Read the model definition and answer for the solid it produces. Units are mm, in the model's axes. Face numbers are marked on the shaded views. Give positions to 0.01 mm unless a question says otherwise; leave off trailing zeros. Loops run counter-clockwise (first coordinate to the right, second up) from the corner with the lowest first, then second, coordinate; pieces in that order, holes last. Notation, with made-up numbers: (49, 59.25) -> (77, 59.25) arc R21 cw to (77, 93.25) -> close; hole circle Ø11 at (86.25, 31.5). An arc over 180 degrees is marked (long way). Return JSON: item names as keys, results as strings. Group by question number.
Autodesk Inventor part; units mm, degrees
ref_plane "YZ Plane" through (0, 0, 0) normal (1, 0, 0) x (0, 1, 0)
ref_plane "XZ Plane" through (0, 0, 0) normal (0, 1, 0) x (-1, 0, 0)
ref_plane "XY Plane" through (0, 0, 0) normal (0, 0, 1) x (1, 0, 0)
sketch "Sketch1" plane through (0, 0, 0) normal (0, 0, 1) x (1, 0, 0)
  line L0 (0, 23.5) -> (3, 23.5)
  line L1 (5, 25.5) -> (5, 29.2)
  line L2 (5, 29.2) -> (10, 29.2)
  line L3 (10, 29.2) -> (10, 31.5)
  line L4 (10, 31.5) -> (0, 31.5)
  line L5 (0, 23.5) -> (0, 39.7331)
  arc A0 (3, 23.5) -> (5, 25.5) centre (3, 25.5) ccw
  line L6 (0, 0) -> (48.7382, 0)
  line L7 (0, 23.5) -> (-3, 23.5)
  line L8 (-5, 25.5) -> (-5, 29.2)
  line L9 (-5, 29.2) -> (-10, 29.2)
  line L10 (-10, 29.2) -> (-10, 31.5)
  line L11 (-10, 31.5) -> (0, 31.5)
  arc A1 (-5, 25.5) -> (-3, 23.5) centre (-3, 25.5) ccw
  dimension "d0" = 2
  dimension "d1" = 47
  dimension "d2" = 63
  dimension "d3" = 58.4
  dimension "d4" = 10
  dimension "d7" = 10
revolve "Revolution1" add sketch "Sketch1" angle 360 about axis through (0, 0, 0) along (1, 0, 0)
chamfer "Fase1" distance 1 angle 45 1 edges at (10, -29.2, 0)
chamfer "Fase2" distance 1 angle 45 1 edges at (-10, -29.2, 0)
properties part number "Plunger_Seal" material "Nylon-6/6"
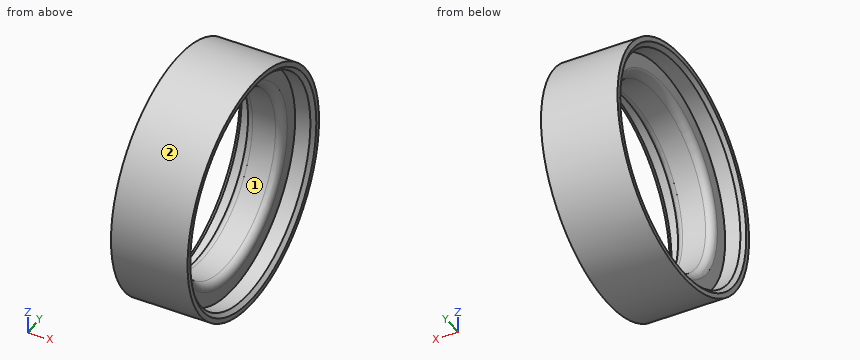
1. Section D-D on x = -7.5 is taken. Determine the outline of the cut face in (y, z), then the cut area to 3 significant figures.
2. Flat-ended cylindrical pins translate along their axes: pin 1 Ø8 at (x, z) = (-7.5, -25) entering from -Y; pin 2 Ø17.5 at (y, z) = (-12.5, -9) entering from +X; pin 3 Ø3 at (x, y) = (-7, -7.5) entering from +Z; pin 4 Ø2 at (y, z) = (-17.5, -14) entering from +X. Find the tip coordinate at first contact, or state that the pin passes through.
3. Determine the mould class of the marked faces 1 and 2 for opening direction Z: pulls with the +Z half, pulls with the -Z half, needs draft (parallel to the pull), parting line crosses it, or undercut.
4. Section A-A on z = 0 is taken. Determine the outline of the cut face in (x, y), then the cut area to 3 significant figures.
5. Section C-C on x = -2 is taken. Determine the outline of the cut face in (y, z).
6. Straight lines are drawn through the part: line 1 (Z direction, x = 7.75, y = 0); line 2 (Y direction, x = -6, z = -1); line 3 (X direction, y = 14, z = -25). For each, find the intervals that lie inside material, in ascending order. Write a range as from..to.
Completed:
{
 "1": {"outline": "circle Ø63 at (0, 0); hole circle Ø58.4 at (0, 0)", "area": "439 mm²"},
 "2": {"pin 1": "stops at y = -23.48", "pin 2": "stops at x = 4.48", "pin 3": "stops at z = 30.92", "pin 4": "passes through"},
 "3": {"face 1": "undercut", "face 2": "parting line crosses it"},
 "4": {"outline": "(-10, -31.5) -> (10, -31.5) -> (10, -30.2) -> (9, -29.2) -> (5, -29.2) -> (5, -25.5) arc R2 ccw to (3, -23.5) -> (-3, -23.5) arc R2 ccw to (-5, -25.5) -> (-5, -29.2) -> (-9, -29.2) -> (-10, -30.2) -> close; (-10, 30.2) -> (-9, 29.2) -> (-5, 29.2) -> (-5, 25.5) arc R2 ccw to (-3, 23.5) -> (3, 23.5) arc R2 ccw to (5, 25.5) -> (5, 29.2) -> (9, 29.2) -> (10, 30.2) -> (10, 31.5) -> (-10, 31.5) -> close", "area": "201 mm²"},
 "5": {"outline": "circle Ø63 at (0, 0); hole circle Ø47 at (0, 0)"},
 "6": {"line 1": "z = -31.5..-29.2, 29.2..31.5", "line 2": "y = -31.48..-29.18, 29.18..31.48", "line 3": "x = -5..5"}
}
